from build123d import *

# Parameters (mm, degrees)
ESQUISSE1_R             = 4
BOSS_EXTRU_1_DEPTH      = 3
ESQUISSE2_R             = 11
BOSS_EXTRU_2_DEPTH      = 2
ESQUISSE4_R             = 1.7
ENL_V_MAT_EXTRU_1_DEPTH = 6
ESQUISSE5_W             = 5.5
ESQUISSE5_H             = 5.5
ENL_V_MAT_EXTRU_2_DEPTH = 1.5


with BuildPart() as part:
    # Esquisse1 → Boss.-Extru.1 (new body)
    with BuildSketch(Plane(origin=(0, 0, 0), x_dir=(1, 0, 0), z_dir=(0, 1, 0))):
        with BuildLine():
            Line((-50.6, 5.969925), (-1.1, 10.944862))
            ThreePointArc((-1.1, 10.944862), (11, 0), (-1.1, -10.944862))
            Line((-1.1, -10.944862), (-50.6, -5.969925))
            ThreePointArc((-50.6, -5.969925), (-56, 0), (-50.6, 5.969925))
        make_face()
        with Locations((-50, 0)):
            Circle(ESQUISSE1_R, mode=Mode.SUBTRACT)
        with Locations((-40, 0)):
            Circle(ESQUISSE1_R, mode=Mode.SUBTRACT)
        with Locations((-30, 0)):
            Circle(ESQUISSE1_R, mode=Mode.SUBTRACT)
        with Locations((-20, 0)):
            Circle(ESQUISSE1_R, mode=Mode.SUBTRACT)
    extrude(amount=BOSS_EXTRU_1_DEPTH)

    # Esquisse2 → Boss.-Extru.2 (add)
    with BuildSketch(Plane(origin=(0, 3, 0), x_dir=(1, 0, 0), z_dir=(0, 1, 0))):
        Circle(ESQUISSE2_R)
    extrude(amount=BOSS_EXTRU_2_DEPTH)

    # Esquisse4 → Enlèv. mat.-Extru.1 (cut, through all)
    with BuildSketch(Plane(origin=(0, 5, 0), x_dir=(1, 0, 0), z_dir=(0, 1, 0))):
        Circle(ESQUISSE4_R)
        with Locations((0, 6)):
            Circle(ESQUISSE4_R)
        with Locations((6, 0)):
            Circle(ESQUISSE4_R)
        with Locations((0, -6)):
            Circle(ESQUISSE4_R)
        with Locations((-6, 0)):
            Circle(ESQUISSE4_R)
    extrude(amount=-ENL_V_MAT_EXTRU_1_DEPTH, mode=Mode.SUBTRACT)

    # Esquisse5 → Enlèv. mat.-Extru.2 (cut)
    with BuildSketch(Plane.XZ):
        Rectangle(ESQUISSE5_W, ESQUISSE5_H)
    extrude(amount=-ENL_V_MAT_EXTRU_2_DEPTH, mode=Mode.SUBTRACT)


solid = part.part
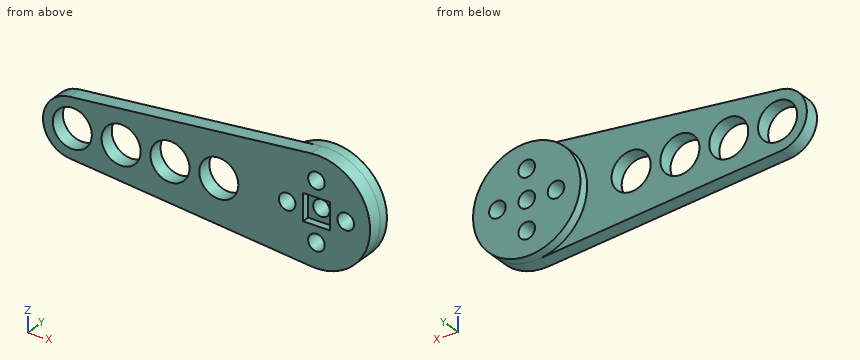
Here's how the part is built. I have some questions about the finished solid (model axes, mm). Round coordinates to 2 decimals unless told otherwise and drop trailing zeros. Write each loop counter-clockwise with the first axis right and the second up, starting at its lowest first coordinate (ties: lowest second). Pieces come first, ordered by that corner, then holes.
1. Suppose I cut it at D-D (x = -9.5). List the corners of the cut face in (y, z) for me.
2. Suppose I cut it at B-B (x = -40). List the corners of the cut face in (y, z) for me, and give its area (3 significant figures).
3. I need wall thicknesses on L1, parallel to Z at x = 0, y = 3.9; L2, parallel to X at y = 0.55, z = 2.25; L3, parallel to X at y = 1.6, z = -3.5. Which ranges of each line are inside material? Lowest first, please.
4. Suppose I cut it at A-A (y = 2.1). State how many separate pieces and enclosed holes the cut face has, and give its area (3 significant figures).
5. Suppose I cut it at C-C (x = -49). List the corners of the cut face in (y, z) for me, and give its area (3 significant figures).
6. Will these pins go through, and if not, where does the flat tip stop? pin 1 Ø1 at (y, z) = (0.5, -7.5) entering from +X; pin 2 Ø13 at (x, z) = (-20, 0) entering from +Y; pin 3 Ø1 at (y, z) = (4, 6.5) entering from -X.
Answer sheet:
1. outline: (0, -10.1) - (3, -10.1) - (3, -5.55) - (5, -5.55) - (5, 5.55) - (3, 5.55) - (3, 10.1) - (0, 10.1) - close
2. outline: (0, -7.04) - (3, -7.04) - (3, -4) - (0, -4) - close; (0, 4) - (3, 4) - (3, 7.04) - (0, 7.04) - close
2. area: 18.2 mm2
3. L1: z = -11 to -7.7, -4.3 to -1.7, 1.7 to 4.3, 7.7 to 11
3. L2: x = -55.56 to -53.31, -46.69 to -43.31, -36.69 to -33.31, -26.69 to -23.31, -16.69 to -2.75, 2.75 to 10.77
3. L3: x = -54.87 to -51.94, -48.06 to -41.94, -38.06 to -31.94, -28.06 to -21.94, -18.06 to 10.43
4. separate pieces: 1
4. enclosed holes: 9
4. area: 854 mm2
5. outline: (0, -6.13) - (3, -6.13) - (3, -3.87) - (0, -3.87) - close; (0, 3.87) - (3, 3.87) - (3, 6.13) - (0, 6.13) - close
5. area: 13.5 mm2
6. pin 1: stops at x = 8.49
6. pin 2: stops at y = 3
6. pin 3: stops at x = -9.22
